Could you check a few things on this model? Use its own coordinates, in mm. A direction names the side the tool comes from. Round coordinates to 2 decimals unless told otherwise and drop trailing zeros. Write each loop counter-clockwise with the first axis right and the second up, starting at its lowest first coordinate (ties: lowest second). Pieces come first, ordered by that corner, then holes. Notation, with made-up numbers: (33.5, 12) - (45.5, 12) arc R29 ccw to (45.5, 46) - close; hole circle Ø8 at (53.25, -8). An arc over 180 degrees is marked (long way). Write each question's results on one line, items separated by ' | '. Start each with the question number.
(1) For P1, Ø3, axis at x = -17, y = 27, coming from the -Z side, with a flat end and sliding along its axis, tell me the tip position at first contact or that it passes through.
(2) Please list where these lines run through material, in increasing order: line 1 (X direction, y = 25, z = -32.4); line 2 (X direction, y = 25.5, z = -20); line 3 (Z direction, x = -8.5, y = 27.5). Write a range as [from, to].
(3) Imagine slicing it at A-A on z = -28.5. Write out the boundary of the cut face in (x, y), then the cut area to 3 significant figures.
(4) Thinking about a two-plate mould opening in Y: for faces 1 (the flat face through (-20, 0, 68)), 2 (the flat face through (-29, 25, -40.5)), 3 (the cylindrical face through (-27.86, 24.52, 32.26)), 4 (the cylindrical face through (-20, 28, -67)), which applies, +Y half, -Y half, draft (parallel to the pull), parting line (faces both ways), or undercut?
(5) Imagine slicing it at B-B on z = 34.5. Write out the boundary of the cut face in (x, y), then the cut area to 3 significant figures.
(6) On a 3-axis mill with a long thin cutter (end or side, diameter ignored), from which of +Z, -Z, +X, -X, +Y, -Y can I reach the whole of each face in a straight line? I mean faces 5 (the cylindrical face through (-20, 29, 66)), 6 (the flat face through (-3.01, 25, -1)), 7 (the cylindrical face through (-27.86, 24.52, -39.76)). Say none if no direction works.
```python
from build123d import *

# Parameters (mm, degrees)
BOSS_EXTRUDE1_DEPTH = 40
CUT_EXTRUDE1_DEPTH  = 10
CUT_EXTRUDE2_START  = -1.5
SKETCH5_R           = 1.25
CUT_EXTRUDE2_DEPTH  = 9


with BuildPart() as part:
    # Sketch1 → Boss-Extrude1 (new body)
    with BuildSketch(Plane(origin=(0, 0, 0), x_dir=(0, 0, -1), z_dir=(1, 0, 0))):
        with BuildLine():
            Line((-63, -30), (63, -30))
            ThreePointArc((63, -30), (66.535533906, -28.535533906), (68, -25))
            Line((68, -25), (68, 25))
            ThreePointArc((68, 25), (66.535533906, 28.535533906), (63, 30))
            Line((63, 30), (-63, 30))
            ThreePointArc((-63, 30), (-66.535533906, 28.535533906), (-68, 25))
            Line((-68, 25), (-68, -25))
            ThreePointArc((-68, -25), (-66.535533906, -28.535533906), (-63, -30))
        make_face()
    extrude(amount=-BOSS_EXTRUDE1_DEPTH)

    # Sketch3 → Cut-Extrude1 (cut)
    with BuildSketch(Plane(origin=(0, 30, 0), x_dir=(1, 0, 0), z_dir=(0, 1, 0))):
        with BuildLine():
            Line((-3.009553383, -37), (-23.009553383, -37))
            Line((-23.009553383, -37), (-23.009553383, -39))
            Line((-23.009553383, -39), (-32.009553383, -39))
            Line((-32.009553383, -39), (-32.009553383, -33))
            Line((-32.009553383, -33), (-8.009553383, -33))
            Line((-8.009553383, -33), (-8.009553383, -4.067313184))
            ThreePointArc((-8.009553383, -4.067313184), (-10.584205762, 0), (-8.009553383, 4.067313184))
            Line((-8.009553383, 4.067313184), (-8.009553383, 33))
            Line((-8.009553383, 33), (-32.009553383, 33))
            Line((-32.009553383, 33), (-32.009553383, 39))
            Line((-32.009553383, 39), (-23.009553383, 39))
            Line((-23.009553383, 39), (-23.009553383, 37))
            Line((-23.009553383, 37), (-3.009553383, 37))
            Line((-3.009553383, 37), (-3.009553383, -37))
        make_face()
    extrude(amount=-CUT_EXTRUDE1_DEPTH, mode=Mode.SUBTRACT)

    # Sketch5 → Cut-Extrude2 (cut)
    with BuildSketch(Plane.XY.offset(-39).offset(CUT_EXTRUDE2_START)):
        with Locations((-29.012566775, 25)):
            Circle(SKETCH5_R)
    cut_extrude2 = extrude(amount=CUT_EXTRUDE2_DEPTH, mode=Mode.SUBTRACT)

    # Mirror1: Cut-Extrude2 across plane
    add(cut_extrude2.mirror(Plane.XY), mode=Mode.SUBTRACT)


solid = part.part
```
Response:
1) P1: z = -67.97
2) line 1: [-40, -30.26], [-27.76, -8.01], [-3.01, 0] | line 2: [-40, -8.01], [-3.01, 0] | line 3: [-67.33, -37], [-33, -3.8], [3.8, 33], [37, 67.33]
3) outline: (-40, -30) - (0, -30) - (0, 30) - (-3.01, 30) - (-3.01, 20) - (-8.01, 20) - (-8.01, 30) - (-40, 30) - close | area: 2,350 mm²
4) face 1: draft | face 2: undercut | face 3: undercut | face 4: +Y half
5) outline: (-40, -30) - (0, -30) - (0, 30) - (-3.01, 30) - (-3.01, 20) - (-32.01, 20) - (-32.01, 30) - (-40, 30) - close | area: 2,110 mm²
6) face 5: +Z, +X, -X, +Y | face 6: +Y | face 7: none
